```python
from build123d import *

# Parameters (mm, degrees)
BOSS_EXTRUDE1_DEPTH = 2.9
SKETCH5_R           = 1.5
CUT_EXTRUDE1_DEPTH  = 13


with BuildPart() as part:
    # Sketch3 → Boss-Extrude1 (new body, symmetric)
    with BuildSketch(Plane.XY):
        with BuildLine():
            Line((-6, -5), (6, -5))
            Line((6, -5), (6, 2))
            ThreePointArc((6, 2), (6.878679656, 4.121320344), (9, 5))
            Line((9, 5), (15, 5))
            Line((15, 5), (15, 3))
            Line((15, 3), (9, 3))
            ThreePointArc((9, 3), (8.292893219, 2.707106781), (8, 2))
            Line((8, 2), (8, -6))
            ThreePointArc((8, -6), (7.707106781, -6.707106781), (7, -7))
            Line((7, -7), (-7, -7))
            ThreePointArc((-7, -7), (-7.707106781, -6.707106781), (-8, -6))
            Line((-8, -6), (-8, 2))
            ThreePointArc((-8, 2), (-8.292893219, 2.707106781), (-9, 3))
            Line((-9, 3), (-15, 3))
            Line((-15, 3), (-15, 5))
            Line((-15, 5), (-9, 5))
            ThreePointArc((-9, 5), (-6.878679656, 4.121320344), (-6, 2))
            Line((-6, 2), (-6, -5))
        make_face()
    extrude(amount=BOSS_EXTRUDE1_DEPTH, both=True)

    # Sketch5 → Cut-Extrude1 (cut, through all)
    with BuildSketch(Plane(origin=(0, 5, 0), x_dir=(1, 0, 0), z_dir=(0, 1, 0))):
        with Locations((12, 0)):
            Circle(SKETCH5_R)
        with Locations((-12, 0)):
            Circle(SKETCH5_R)
    extrude(amount=-CUT_EXTRUDE1_DEPTH, mode=Mode.SUBTRACT)


solid = part.part
```
The model under review builds one solid part; all positions refer to its coordinate system, in mm. A direction names the side the tool comes from. Coordinates: 2 decimals unless noted, no trailing zeros. Loops run counter-clockwise (first coordinate to the right, second up) from the corner with the lowest first, then second, coordinate; pieces in that order, holes last. Notation, with made-up numbers: (36.5, 15) -> (91.5, 15) arc R4 cw to (91.5, 22) -> close; hole circle Ø5 at (87.5, 20.25). An arc over 180 degrees is marked (long way). Answer as CSV lines item,"result".
Item 1: Machinability: for faces 5 (the flat face through (8, -2, 0)), 6 (the flat face through (-10.6, 3, 1.3)), 7 (the flat face through (10.6, 5, 1.3)), 8 (the flat face through (0, -7, 0)), 9 (the cylindrical face through (6.86, 4.1, 0.04)), which of the approach directions +Z, -Z, +X, -X, +Y, -Y give a long, thin tool a straight path to every point of the face, cutting with its end or side? Answer none if there is none.
Results below:
face 5,"+Z, -Z, +X, -Y"
face 6,"+Z, -Z, -X, -Y"
face 7,"+Z, -Z, +X, -X, +Y"
face 8,"+Z, -Z, +X, -X, -Y"
face 9,"+Z, -Z, +Y"
Item 2: For L1, parallel to Z at x = 12, y = 4; L2, parallel to X at y = -2.25, z = -2.4; L3, parallel to X at y = 3.25, z = 0.75, list the stretches that pass through material, from the lowest coordinate up.
Results below:
L1,"z = -2.9 to -1.5, 1.5 to 2.9"
L2,"x = -8 to -6, 6 to 8"
L3,"x = -15 to -13.3, -10.7 to -6.27, 6.27 to 10.7, 13.3 to 15"
Item 3: Take a section at A-A, the plane x = 12. State the section outline as (y, z) points, and give its area (3 significant figures).
Results below:
outline,"(3, -2.9) -> (5, -2.9) -> (5, -1.5) -> (3, -1.5) -> close; (3, 1.5) -> (5, 1.5) -> (5, 2.9) -> (3, 2.9) -> close"
area,"5.60 mm2"
Item 4: Draft analysis for pull direction X (two halves, no side actions). For faces 1 (the cylindrical face through (-6.9, 4.14, 0.04)), 2 (the flat face through (1.2, -5.4, 2.9)), 3 (the flat face through (-15, 4, 0)), 4 (the flat face through (-6, -1, 0)), state which applies: +X half, -X half, draft (parallel to the pull), parting line (faces both ways), or undercut.
Results below:
face 1,"undercut"
face 2,"draft"
face 3,"-X half"
face 4,"undercut"
Item 5: Take a section at C-C, the plane y = -4. State the section outline as (x, z) points.
Results below:
outline,"(-8, -2.9) -> (-6, -2.9) -> (-6, 2.9) -> (-8, 2.9) -> close; (6, -2.9) -> (8, -2.9) -> (8, 2.9) -> (6, 2.9) -> close"
Item 6: Take a section at D-D, the plane z = 2.5. State the section outline as (x, y) points.
Results below:
outline,"(-15, 3) -> (-9, 3) arc R1 cw to (-8, 2) -> (-8, -6) arc R1 ccw to (-7, -7) -> (7, -7) arc R1 ccw to (8, -6) -> (8, 2) arc R1 cw to (9, 3) -> (15, 3) -> (15, 5) -> (9, 5) arc R3 ccw to (6, 2) -> (6, -5) -> (-6, -5) -> (-6, 2) arc R3 ccw to (-9, 5) -> (-15, 5) -> close"
Item 7: Insertion check: pin 1 (4 mm diameter, centred on x = 10.5, y = -4, fed in from -Z); pin 2 (3 mm diameter, centred on y = -1.5, z = 0.5, fed in from +X); pin 3 (1.5 mm diameter, centred on x = 1, z = 0, fed in from +Y); pin 4 (1.7 mm diameter, centred on x = 11.5, z = 1, fed in from -Y). Each pin has a flat end and moves straight along its axis. Give the tip position at first contact, or say it passes through.
Results below:
pin 1,"passes through"
pin 2,"stops at x = 8"
pin 3,"stops at y = -5"
pin 4,"stops at y = 3"
Item 8: Take a section at B-B, the plane z = 0. State the section outline as (x, y) points, and give its area (3 significant figures).
Results below:
outline,"(-15, 3) -> (-13.5, 3) -> (-13.5, 5) -> (-15, 5) -> close; (-10.5, 3) -> (-9, 3) arc R1 cw to (-8, 2) -> (-8, -6) arc R1 ccw to (-7, -7) -> (7, -7) arc R1 ccw to (8, -6) -> (8, 2) arc R1 cw to (9, 3) -> (10.5, 3) -> (10.5, 5) -> (9, 5) arc R3 ccw to (6, 2) -> (6, -5) -> (-6, -5) -> (-6, 2) arc R3 ccw to (-9, 5) -> (-10.5, 5) -> close; (13.5, 3) -> (15, 3) -> (15, 5) -> (13.5, 5) -> close"
area,"84.1 mm2"
